```python
from build123d import *

# Parameters (mm, degrees)
BOSS_EXTRUDE1_DEPTH = 5
SCALE1_SCALE        = 0.15


with BuildPart() as part:
    # Sketch3 → Boss-Extrude1 (new body)
    with BuildSketch(Plane(origin=(0, 0, 0), x_dir=(1, 0, 0), z_dir=(0, 1, 0))):
        Polygon((-612.771529665, 336.297556136), (-510.771529665, 336.297556136), (-421.771529665, 247.297556136), (-421.771529665, 145.297556136), (-510.771529665, 56.297556136), (-612.771529665, 56.297556136), (-701.771529665, 145.297556136), (-701.771529665, 247.297556136), align=None)
    extrude(amount=BOSS_EXTRUDE1_DEPTH)


with BuildPart() as part_1:
    # Scale1: scaled about (-561.771529665, 2.5, -196.297556136)
    add(part.part.scale(SCALE1_SCALE).moved(Location((-477.505800215, 2.125, -166.852922716))))


solid = part_1.part
```
Here's how the part is built. I have some questions about the finished solid (model axes, mm). Coordinates: 2 decimals unless noted, no trailing zeros. Write each loop counter-clockwise with the first axis right and the second up, starting at its lowest first coordinate (ties: lowest second). Pieces come first, ordered by that corner, then holes. Notation, with made-up numbers: M -8,70 L 20,70 A13 cw 20,77 Z; hole C 2.5,36 d6. An arc over 180 degrees is marked long. Answer as CSV lines item,"result". Start each with the question number.
Q1. If we mould it in two halves opening along Z, with no side actions, what happens to faces 1 (the flat face through (-561, 2.875, -197)), 2 (the flat face through (-576.19, 2.49, -210.53)), 3 (the flat face through (-547.35, 2.49, -182.07))? For each: pulls with the +Z half, pulls with the -Z half, needs draft (parallel to the pull), parting line crosses it, or undercut.
Q2. Suppose I cut it at A-A, the plane y = 2.6. List the corners of the cut face in (x, z) for me.
Q3. Suppose I cut it at B-B, the plane z = -181. List the corners of the cut face in (x, y) for me (3 decimals).
Q4. I need wall thicknesses on probe 1 along X at (y, z) = (2.8, -206); probe 2 along X at (y, z) = (2.25, -183); probe 3 along Z at (x, y) = (-543, 2.75). Which ranges of each line are inside material? Lowest first, please. Write a range as [from, to].
Q5. Suppose I cut it at C-C, the plane x = -575. List the corners of the cut face in (y, z) for me (3 decimals).
Entries:
1,face 1,"needs draft"
1,face 2,"pulls with the -Z half"
1,face 3,"pulls with the +Z half"
2,outline,"M -582.77,-203.95 L -569.42,-217.3 L -554.12,-217.3 L -540.77,-203.95 L -540.77,-188.65 L -554.12,-175.3 L -569.42,-175.3 L -582.77,-188.65 Z"
3,outline,"M -575.124,2.125 L -548.419,2.125 L -548.419,2.875 L -575.124,2.875 Z"
4,probe 1,"x = [-580.72, -542.82]"
4,probe 2,"x = [-577.12, -546.42]"
4,probe 3,"z = [-206.18, -186.42]"
5,outline,"M 2.125,-211.719 L 2.875,-211.719 L 2.875,-180.876 L 2.125,-180.876 Z"
